Build history of the part. All positions in model axes, mm. Face numbers are marked on the shaded views. Give positions to 0.01 mm unless a question says otherwise; leave off trailing zeros. Write each loop counter-clockwise with the first axis right and the second up, starting at its lowest first coordinate (ties: lowest second). Pieces come first, ordered by that corner, then holes. Notation, with made-up numbers: M 86,66 L 143,66 A6 cw 143,71 Z; hole C 18,64 d4. An arc over 180 degrees is marked long. Return JSON: item names as keys, results as strings. Group by question number.
Q1. Band-saw the part on C-C, the plane x = 88.5. Give the cut face in (y, z).
Q2. Band-saw the part on D-D, the plane x = 150. Give the cut face in (y, z), then the cut area to 3 significant figures.
Q3. Band-saw the part on B-B, the plane y = 36.5. Give the cut face in (x, z), then the cut area to 3 significant figures.
Q4. Flat gauge pin, fed straight in: pin 1 Ø8 at (x, y) = (150, 90) entering from -Z. Where does the tip first touch, or does it go through?
Q5. Band-saw the part on A-A, the plane z = 15. Give the cut face in (x, y), then the cut area to 3 significant figures.
Q6. Wall check: probe 1 along X at (y, z) = (90, 6); probe 2 along Y at (x, z) = (110, 15); probe 3 along Y at (x, z) = (20.5, 15.5). Give the ranges that are in metal, low to high.
Q7. Pull direction X, two halves, no side cores. Call the marked faces 1, 2, 3 and 4: +X half, -X half, draft (parallel to the pull), parting line (faces both ways), or undercut.
from build123d import *

# Parameters (mm, degrees)
F0_W     = 400
F0_H     = 200
F1_DEPTH = 50
F2_W     = 360
F2_H     = 160
F3_DEPTH = 25
F4_R     = 5
F5_DEPTH = 20


with BuildPart() as f1:
    # F0 (on Top) → F1 (new body)
    with BuildSketch(Plane.XY):
        Rectangle(F0_W, F0_H)
    extrude(amount=F1_DEPTH)

    # F2 (on face) → F3 (cut)
    with BuildSketch(Plane(origin=(0, 0, 0), x_dir=(1, 0, 0), z_dir=(0, 0, -1))):
        Rectangle(F2_W, F2_H)
    extrude(amount=-F3_DEPTH, mode=Mode.SUBTRACT)

    # F4 (on face) → F5 (cut)
    with BuildSketch(Plane(origin=(0, 0, 0), x_dir=(1, 0, 0), z_dir=(0, 0, -1))):
        with Locations((-150, -90)):
            Circle(F4_R)
        with Locations((-110, -90)):
            Circle(F4_R)
        with Locations((110, -90)):
            Circle(F4_R)
        with Locations((150, -90)):
            Circle(F4_R)
    extrude(amount=-F5_DEPTH, mode=Mode.SUBTRACT)


solid = f1.part
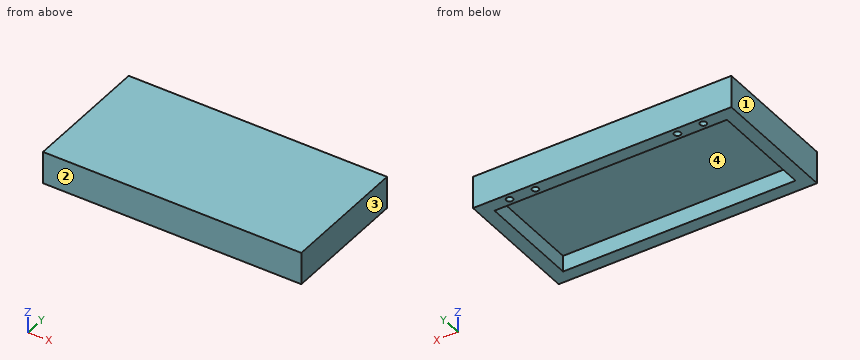
From the geometry:
{
 "1": {"outline": "M -100,0 L -80,0 L -80,25 L 80,25 L 80,0 L 100,0 L 100,50 L -100,50 Z"},
 "2": {"outline": "M -100,0 L -80,0 L -80,25 L 80,25 L 80,0 L 85,0 L 85,20 L 95,20 L 95,0 L 100,0 L 100,50 L -100,50 Z", "area": "5,800 mm^2"},
 "3": {"outline": "M -200,0 L -180,0 L -180,25 L 180,25 L 180,0 L 200,0 L 200,50 L -200,50 Z", "area": "11,000 mm^2"},
 "4": {"pin 1": "stops at z = 20"},
 "5": {"outline": "M -200,-100 L 200,-100 L 200,100 L -200,100 Z; hole M -180,-80 L 180,-80 L 180,80 L -180,80 Z; hole C -150,90 d10; hole C -110,90 d10; hole C 110,90 d10; hole C 150,90 d10", "area": "22,100 mm^2"},
 "6": {"probe 1": "x = -200 to -155, -145 to -115, -105 to 105, 115 to 145, 155 to 200", "probe 2": "y = -100 to -80, 80 to 85, 95 to 100", "probe 3": "y = -100 to -80, 80 to 100"},
 "7": {"face 1": "-X half", "face 2": "draft", "face 3": "+X half", "face 4": "undercut"}
}
